```python
from build123d import *

# Parameters (mm, degrees)
BOSS_EXTRU_1_DEPTH = 3
CONG_1_R           = 0.2
BOSS_EXTRU_2_DEPTH = 5.565397746


with BuildPart() as part:
    # Esquisse1 → Boss.-Extru.1 (new body)
    with BuildSketch(Plane.XY):
        with BuildLine():
            Line((-2.5, -3), (2.5, -3))
            ThreePointArc((2.5, -3), (2.853553391, -2.853553391), (3, -2.5))
            Line((3, -2.5), (3, 2.5))
            ThreePointArc((3, 2.5), (2.853553391, 2.853553391), (2.5, 3))
            Line((2.5, 3), (-2.5, 3))
            ThreePointArc((-2.5, 3), (-2.853553391, 2.853553391), (-3, 2.5))
            Line((-3, 2.5), (-3, -2.5))
            ThreePointArc((-3, -2.5), (-2.853553391, -2.853553391), (-2.5, -3))
        make_face()
    extrude(amount=BOSS_EXTRU_1_DEPTH)

    # Congé1
    cong_1_edges = [part.edges().sort_by_distance(p)[0] for p in [
        (2.853553391, -2.853553391, 3),
        (3, 0, 3),
        (2.853553391, 2.853553391, 3),
        (0, 3, 3),
        (-2.853553391, 2.853553391, 3),
        (-3, 0, 3),
        (-2.853553391, -2.853553391, 3),
        (0, -3, 3),
    ]]
    fillet(cong_1_edges, radius=CONG_1_R)

    # Esquisse2 → Boss.-Extru.2 (add)
    with BuildSketch(Plane.XY):
        with BuildLine():
            Line((-3.5, -4), (3.5, -4))
            ThreePointArc((3.5, -4), (3.853553391, -3.853553391), (4, -3.5))
            Line((4, -3.5), (4, 3.5))
            ThreePointArc((4, 3.5), (3.853553391, 3.853553391), (3.5, 4))
            Line((3.5, 4), (-3.5, 4))
            ThreePointArc((-3.5, 4), (-3.853553391, 3.853553391), (-4, 3.5))
            Line((-4, 3.5), (-4, -3.5))
            ThreePointArc((-4, -3.5), (-3.853553391, -3.853553391), (-3.5, -4))
        make_face()
    extrude(amount=-BOSS_EXTRU_2_DEPTH)


solid = part.part
```
Verification items for the finished model (mm, model axes). A direction names the side the tool comes from. Coordinates: 2 decimals unless noted, no trailing zeros. Write each loop counter-clockwise with the first axis right and the second up, starting at its lowest first coordinate (ties: lowest second). Pieces come first, ordered by that corner, then holes. Notation, with made-up numbers: M 60,-5.75 L 66,-5.75 A14 ccw 66,8.25 Z; hole C 39.25,-15.5 d6. An arc over 180 degrees is marked long. One line per item, written item: value.
Item 1: Scan lines: line 1 along Z through (x, y) = (3.5, 0); line 2 along X through (y, z) = (0.5, 2.25). Record each from-to range of solid material in increasing order.
Check sheet entries:
line 1: z = -5.57 to 0
line 2: x = -3 to 3
Item 2: Section check A-A, the plane x = -1.5. Record the boundary of the cut face in (y, z), plus the area to 3 significant figures.
Check sheet entries:
outline: M -4,-5.57 L 4,-5.57 L 4,0 L 3,0 L 3,2.8 A0.2 ccw 2.8,3 L -2.8,3 A0.2 ccw -3,2.8 L -3,0 L -4,0 Z
area: 62.5 mm^2
Item 3: Section check D-D, the plane x = 3.25. Record the boundary of the cut face in (y, z).
Check sheet entries:
outline: M -4,-5.57 L 4,-5.57 L 4,0 L -4,0 Z
Item 4: Gauge pin test, flat ends, axial feed: pin 1 Ø0.8 at (x, z) = (0.5, 2) entering from -Y; pin 2 Ø1.4 at (x, z) = (-0.5, 2) entering from +Y. Record the tip position at first contact, or that the pin passes through.
Check sheet entries:
pin 1: stops at y = -3
pin 2: stops at y = 3
Item 5: Access from +Z, -Z, +X, -X, +Y, -Y to the whole of each face (thin tool, end or side, straight path). Record for faces 1 (the flat face through (3, 0, 1)), 2 (the flat face through (-3, 0, 1)), 3 (the flat face through (0, -3, 1)).
Check sheet entries:
face 1: +Z, +X, +Y, -Y
face 2: +Z, -X, +Y, -Y
face 3: +Z, +X, -X, -Y
Item 6: Section check C-C, the plane z = 0.25. Record the boundary of the cut face in (x, y), plus the area to 3 significant figures.
Check sheet entries:
outline: M -3,-2.5 A0.5 ccw -2.5,-3 L 2.5,-3 A0.5 ccw 3,-2.5 L 3,2.5 A0.5 ccw 2.5,3 L -2.5,3 A0.5 ccw -3,2.5 Z
area: 35.8 mm^2
